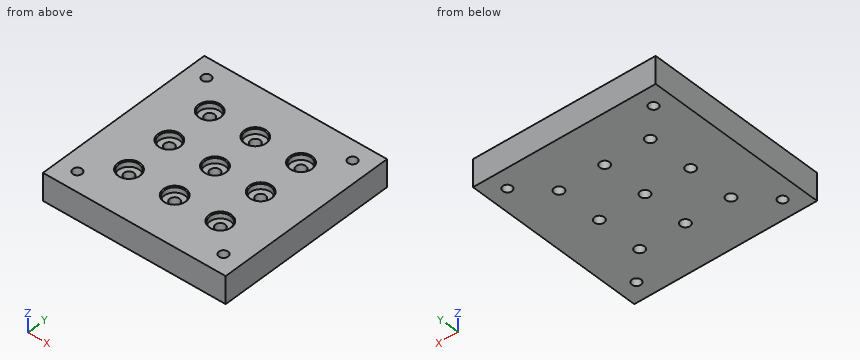
from build123d import *

# Parameters (mm, degrees)
SKETCH2_W                       = 127
SKETCH2_H                       = 127
BOSS_EXTRUDE1_DEPTH             = 19.05
LPATTERN1_COUNT                 = 2
LPATTERN1_PITCH                 = 31.75
LPATTERN1_COL_COUNT             = 2
LPATTERN1_COL_PITCH             = 31.75
LPATTERN2_COUNT                 = 2
LPATTERN2_PITCH                 = 31.75
LPATTERN2_COL_COUNT             = 2
LPATTERN2_COL_PITCH             = 31.75
F_1_4_0_25_DIAMETER_HOLE1_D     = 6.35
F_1_4_0_25_DIAMETER_HOLE1_DEPTH = 59.944
F_1_4_0_25_DIAMETER_HOLE1_TIP   = 1.907732465


with BuildPart() as part:
    # Sketch2 → Boss-Extrude1 (new body)
    with BuildSketch(Plane.XY):
        Rectangle(SKETCH2_W, SKETCH2_H)
    extrude(amount=BOSS_EXTRUDE1_DEPTH)

    # Sketch5 → CBORE for 1/4 Binding Head Machine Screw1 (revolve, cut)
    with BuildSketch(Plane(origin=(0, 0, 19.05), x_dir=(0, -1, 0), z_dir=(1, 0, 0))):
        Polygon((0, 0), (0, 19.05), (3.3782, 19.05), (3.3782, 4.191), (7.14375, 4.191), (7.14375, 0.635), (7.77875, 0), align=None)
    cbore_for_1_4_binding_head_machine_screw = revolve(axis=Axis((0, 0, 25.4), (0, 0, -1)), mode=Mode.SUBTRACT)

    # LPattern1: CBORE for 1/4 Binding Head Machine Screw1 ×2
    with Locations(*[(i * LPATTERN1_PITCH, 0, 0) for i in range(1, LPATTERN1_COUNT)]):
        add(cbore_for_1_4_binding_head_machine_screw, mode=Mode.SUBTRACT)

    # LPattern1 col: CBORE for 1/4 Binding Head Machine Screw1 ×2
    with Locations(*[(-i * LPATTERN1_COL_PITCH, 0, 0) for i in range(1, LPATTERN1_COL_COUNT)]):
        add(cbore_for_1_4_binding_head_machine_screw, mode=Mode.SUBTRACT)

    # LPattern2: CBORE for 1/4 Binding Head Machine Screw1 ×2
    with Locations(*[(0, -i * LPATTERN2_PITCH, 0) for i in range(1, LPATTERN2_COUNT)]):
        add(cbore_for_1_4_binding_head_machine_screw, mode=Mode.SUBTRACT)

    # LPattern2 copy 1 sketch → LPattern2 copy 1 (revolve, cut)
    with BuildSketch(Plane(origin=(31.75, -31.75, 19.05), x_dir=(0, -1, 0), z_dir=(1, 0, 0))):
        Polygon((0, 0), (0, 19.05), (3.3782, 19.05), (3.3782, 4.191), (7.14375, 4.191), (7.14375, 0.635), (7.77875, 0), align=None)
    revolve(axis=Axis((31.75, -31.75, 25.4), (0, 0, -1)), mode=Mode.SUBTRACT)

    # LPattern2 copy 2 sketch → LPattern2 copy 2 (revolve, cut)
    with BuildSketch(Plane(origin=(-31.75, -31.75, 19.05), x_dir=(0, -1, 0), z_dir=(1, 0, 0))):
        Polygon((0, 0), (0, 19.05), (3.3782, 19.05), (3.3782, 4.191), (7.14375, 4.191), (7.14375, 0.635), (7.77875, 0), align=None)
    revolve(axis=Axis((-31.75, -31.75, 25.4), (0, 0, -1)), mode=Mode.SUBTRACT)

    # LPattern2 col: CBORE for 1/4 Binding Head Machine Screw1 ×2
    with Locations(*[(0, i * LPATTERN2_COL_PITCH, 0) for i in range(1, LPATTERN2_COL_COUNT)]):
        add(cbore_for_1_4_binding_head_machine_screw, mode=Mode.SUBTRACT)

    # LPattern2 col copy 1 sketch → LPattern2 col copy 1 (revolve, cut)
    with BuildSketch(Plane(origin=(31.75, 31.75, 19.05), x_dir=(0, -1, 0), z_dir=(1, 0, 0))):
        Polygon((0, 0), (0, 19.05), (3.3782, 19.05), (3.3782, 4.191), (7.14375, 4.191), (7.14375, 0.635), (7.77875, 0), align=None)
    revolve(axis=Axis((31.75, 31.75, 25.4), (0, 0, -1)), mode=Mode.SUBTRACT)

    # LPattern2 col copy 2 sketch → LPattern2 col copy 2 (revolve, cut)
    with BuildSketch(Plane(origin=(-31.75, 31.75, 19.05), x_dir=(0, -1, 0), z_dir=(1, 0, 0))):
        Polygon((0, 0), (0, 19.05), (3.3782, 19.05), (3.3782, 4.191), (7.14375, 4.191), (7.14375, 0.635), (7.77875, 0), align=None)
    revolve(axis=Axis((-31.75, 31.75, 25.4), (0, 0, -1)), mode=Mode.SUBTRACT)

    # 1/4 (0.25) Diameter Hole1
    with Locations(Plane.XY.offset(19.05)):
        with Locations((-50.8, 50.8), (50.8, 50.8), (50.8, -50.8), (-50.8, -50.8)):
            Hole(F_1_4_0_25_DIAMETER_HOLE1_D / 2, depth=F_1_4_0_25_DIAMETER_HOLE1_DEPTH)
            with Locations((0, 0, -(F_1_4_0_25_DIAMETER_HOLE1_DEPTH + F_1_4_0_25_DIAMETER_HOLE1_TIP / 2))):  # 118° drill point
                Cone(0, F_1_4_0_25_DIAMETER_HOLE1_D / 2, F_1_4_0_25_DIAMETER_HOLE1_TIP, mode=Mode.SUBTRACT)


solid = part.part
Work out the finished part from the listing and answer in its coordinate system (mm). Give positions to 0.01 mm unless a question says otherwise; leave off trailing zeros. Loops run counter-clockwise (first coordinate to the right, second up) from the corner with the lowest first, then second, coordinate; pieces in that order, holes last. Notation, with made-up numbers: (2, 52) - (10, 52) arc R29 ccw to (10, 76) - close; hole circle Ø10 at (13, 63). An arc over 180 degrees is marked (long way). Answer in a Markdown table with one row per item. Add a question column.
Q1. Consider line 1 along Y through (x, z) = (-31.75, 5.75); line 2 along X through (y, z) = (31.75, 16.1). Determine where each line is inside the solid, lowest interval first.
Q2. The part is cut by section A-A (x = 31.75). State how many separate pieces and enclosed holes the cut face has, and give its area (3 significant figures).
Q3. Each of these flat-tipped pins is pushed along its axis until it touches: P1, Ø9, axis at x = 31.75, y = -31.75, coming from the +Z side; P2, Ø11.5, axis at x = 32.5, y = -30.5, coming from the +Z side. Where does it stop, or does it pass through?
Q4. The part is cut by section D-D (x = 50.8). Determine the outline of the cut face in (y, z) (3 decimals).
Solution:
| question | item | result |
|---|---|---|
| 1 | line 1 | y = -63.5 to -35.13, -28.37 to -3.38, 3.38 to 28.37, 35.13 to 63.5 |
| 1 | line 2 | x = -63.5 to -38.89, -24.61 to -7.14, 7.14 to 24.61, 38.89 to 63.5 |
| 2 | separate pieces | 4 |
| 2 | enclosed holes | 0 |
| 2 | area | 1,940 mm² |
| 3 | P1 | stops at z = 14.86 |
| 3 | P2 | stops at z = 18.48 |
| 4 | outline | (-63.5, 0) - (-53.975, 0) - (-53.975, 19.05) - (-63.5, 19.05) - close; (-47.625, 0) - (47.625, 0) - (47.625, 19.05) - (-47.625, 19.05) - close; (53.975, 0) - (63.5, 0) - (63.5, 19.05) - (53.975, 19.05) - close |
